```python
from build123d import *

# Parameters (mm, degrees)
F0_R     = 50
F1_DEPTH = 20
F2_R     = 45
F3_DEPTH = 15
F5_DEPTH = 25


with BuildPart() as f1:
    # F0 (on Top) → F1 (new body)
    with BuildSketch(Plane.XY):
        Circle(F0_R)
    extrude(amount=F1_DEPTH)

    # F2 (on face) → F3 (cut)
    with BuildSketch(Plane.XY.offset(20)):
        Circle(F2_R)
    extrude(amount=-F3_DEPTH, mode=Mode.SUBTRACT)

    # F4 (on face) → F5 (join)
    with BuildSketch(Plane.XY.offset(5)):
        with BuildLine():
            ThreePointArc((0, 35), (-6.077686, 34.468271), (-11.970705, 32.889242))
            Line((-11.970705, 32.889242), (-8.550504, 23.492316))
            ThreePointArc((-8.550504, 23.492316), (-4.341204, 24.620194), (0, 25))
            Line((0, 25), (0, 35))
        make_face()
        with BuildLine():
            ThreePointArc((-30.310889, -17.5), (-26.811556, -22.497566), (-22.497566, -26.811556))
            Line((-22.497566, -26.811556), (-16.06969, -19.151111))
            ThreePointArc((-16.06969, -19.151111), (-19.151111, -16.06969), (-21.650635, -12.5))
            Line((-21.650635, -12.5), (-30.310889, -17.5))
        make_face()
        with BuildLine():
            ThreePointArc((30.310889, -17.5), (32.889242, -11.970705), (34.468271, -6.077686))
            Line((34.468271, -6.077686), (24.620194, -4.341204))
            ThreePointArc((24.620194, -4.341204), (23.492316, -8.550504), (21.650635, -12.5))
            Line((21.650635, -12.5), (30.310889, -17.5))
        make_face()
    extrude(amount=F5_DEPTH)


solid = f1.part
```
Build history of the part. All positions in model axes, mm. A direction names the side the tool comes from. Round coordinates to 2 decimals unless told otherwise and drop trailing zeros. Write each loop counter-clockwise with the first axis right and the second up, starting at its lowest first coordinate (ties: lowest second). Pieces come first, ordered by that corner, then holes. Notation, with made-up numbers: (15.5, -16.5) - (65.5, -16.5) arc R6 cw to (65.5, -9.5) - close; hole circle Ø9 at (84, 11.25). An arc over 180 degrees is marked (long way). Write each question's results on one line, items separated by ' | '. Start each with the question number.
Item 1: Saw through at A-A (z = 18.5). Write the cut outline in (x, y).
Item 2: Saw through at B-B (y = 0). Write the cut outline in (x, z), and give its area (3 significant figures).
Item 3: Drop flat-ended pins along their axis: P1, Ø2, axis at x = 13, y = 31.5, coming from the +Z side; P2, Ø2, axis at y = -19.5, z = 26, coming from the +X side; P3, Ø3, axis at y = 28.5, z = 8, coming from the +X side. Give the stop position or say it passes through.
Item 4: Which spindle directions (+Z, -Z, +X, -X, +Y, -Y) get a long thin tool onto all of the face, cutting with end or side? Do faces 5 (the face through (-1, 1, 0)), 6 (the face through (25.92, -14.965, 17.325)). Say none if no direction does.
Item 5: Saw through at C-C (x = -33). Write the cut outline in (y, z).
Item 6: Saw through at D-D (x = 32). Write the cut outline in (y, z), and give its area (3 significant figures).
Item 7: Mould opens along X. For faces 1 (the face through (32.86, -12.05, 17.32)), 2 (the face through (47.69, 15.02, 9.86)), 3 (the face through (-19.11, -16.12, 17.32)), 4 (the face through (-5, 29, 30)) say: pulls with the +X half, pulls with the -X half, needs draft (parallel to the pull), parting line crosses it, or undercut.
Item 8: Wall check: L1, parallel to Y at x = -28, z = 11.5; L2, parallel to X at y = -16.5, z = 17.75; L3, parallel to Y at x = -17.5, z = 5.5. Give the ranges that are in metal, low to high. Write a range as [from, to].
Results are:
1) outline: circle Ø100 at (0, 0); (-30.31, -17.5) arc R35 ccw to (-22.5, -26.81) - (-16.07, -19.15) arc R25 cw to (-21.65, -12.5) - close; (-11.97, 32.89) - (-8.55, 23.49) arc R25 cw to (0, 25) - (0, 35) arc R35 ccw to start; (21.65, -12.5) - (30.31, -17.5) arc R35 ccw to (34.47, -6.08) - (24.62, -4.34) arc R25 cw to start; hole circle Ø90 at (0, 0)
2) outline: (-50, 0) - (50, 0) - (50, 20) - (45, 20) - (45, 5) - (-45, 5) - (-45, 20) - (-50, 20) - close | area: 650 mm²
3) P1: stops at z = 5 | P2: stops at x = -16.07 | P3: stops at x = 42.08
4) face 5: -Z, +X, -X, +Y, -Y | face 6: +Z
5) outline: (-37.56, 0) - (37.56, 0) - (37.56, 20) - (30.59, 20) - (30.59, 5) - (-30.59, 5) - (-30.59, 20) - (-37.56, 20) - close
6) outline: (-38.42, 0) - (38.42, 0) - (38.42, 20) - (31.64, 20) - (31.64, 5) - (-5.64, 5) - (-5.64, 30) - (-14.18, 30) - (-14.18, 5) - (-31.64, 5) - (-31.64, 20) - (-38.42, 20) - close | area: 801 mm²
7) face 1: undercut | face 2: parting line crosses it | face 3: undercut | face 4: needs draft
8) L1: y = [-41.42, -35.23], [-21, -16.17], [35.23, 41.42] | L2: x = [-47.2, -41.87], [-28.58, -18.78], [28.58, 30.87], [41.87, 47.2] | L3: y = [-46.84, -41.46], [-20.86, -17.85], [41.46, 46.84]
